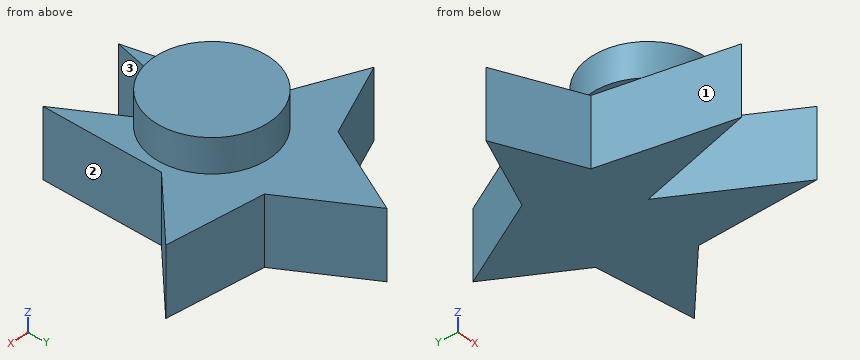
from build123d import *

# Parameters (mm, degrees)
F1_DEPTH = 35.306
F2_R     = 29.733819
F3_DEPTH = 17.526


with BuildPart() as f1:
    # F0 (on Top) → F1 (new body)
    with BuildSketch(Plane.XY):
        Polygon((-6.834473, 83.489791), (-29.494941, 37.89553), (-68.213977, 21.260617), (-28.555268, 3.504229), (-13.849725, -60.445834), (0, 0), (34.043796, -55.656485), (34.043796, 5.008644), (66.349685, 36.453225), (17.759997, 43.004174), align=None)
    extrude(amount=-F1_DEPTH)

    # F2 (on Top) → F3 (join)
    with BuildSketch(Plane.XY):
        Circle(F2_R)
    extrude(amount=F3_DEPTH)


solid = f1.part
Can you work these out from the model? Positions are in its coordinate system, mm. Face numbers are marked on the shaded views. A direction names the side the tool comes from. Give positions to 0.01 mm unless a question says otherwise; leave off trailing zeros. Loops run counter-clockwise (first coordinate to the right, second up) from the corner with the lowest first, then second, coordinate; pieces in that order, holes last. Notation, with made-up numbers: (46.5, -24.75) -> (50.5, -24.75) arc R17 ccw to (50.5, 5.25) -> close; hole circle Ø10 at (54, 78). An arc over 180 degrees is marked (long way). Return JSON: item names as keys, results as strings.
Q1. On a 3-axis mill with a long thin cutter (end or side, diameter ignored), from which of +Z, -Z, +X, -X, +Y, -Y can I reach the whole of each face in a straight line? I mean the marked faces 1, 2 and 3. Say none if no direction works.
Checks:
{"face 1": "-Z, -X, -Y", "face 2": "+Z, -Z, +X, -Y", "face 3": "-Z, -Y"}
Q2. I want a section at B-B, the plane y = -12. List the corners of the cut face in (x, z) for me.
Checks:
{"outline": "(-27.2, 0) -> (-24.99, 0) -> (-24.99, -35.31) -> (-2.75, -35.31) -> (-2.75, 0) -> (7.34, 0) -> (7.34, -35.31) -> (34.04, -35.31) -> (34.04, 0) -> (27.2, 0) -> (27.2, 17.53) -> (-27.2, 17.53) -> close"}
Q3. I need wall thicknesses on probe 1 along Z at (x, y) = (-17.5, 58); probe 2 along X at (y, z) = (-5, -20); probe 3 along Y at (x, z) = (0, 8). Which ranges of each line are inside material? Lowest first, please.
Checks:
{"probe 1": "z = -35.31 to 0", "probe 2": "x = -26.6 to -1.15, 3.06 to 34.04", "probe 3": "y = -29.73 to 29.73"}
Q4. For pin 1 Ø1 at (y, z) = (54, -21.5) entering from +X; pin 2 Ø4 at (y, z) = (-25.5, -7) entering from -X; pin 3 Ø3 at (x, z) = (-11, -26.5) entering from +Y, each with a flat end and sliding along its axis, tell me the tip position at first contact or that it passes through.
Checks:
{"pin 1": "stops at x = 11.38", "pin 2": "stops at x = -22.35", "pin 3": "stops at y = 78.13"}
Q5. I want a section at D-D, the plane y = -36. List the corners of the cut face in (x, z) for me, then the cut area to 3 significant figures.
Checks:
{"outline": "(-19.47, -35.31) -> (-8.25, -35.31) -> (-8.25, 0) -> (-19.47, 0) -> close; (22.02, -35.31) -> (34.04, -35.31) -> (34.04, 0) -> (22.02, 0) -> close", "area": "821 mm2"}
Q6. I want a section at C-C, the plane x = -10. List the corners of the cut face in (y, z) for me, then the cut area to 3 significant figures.
Checks:
{"outline": "(-43.64, -35.31) -> (77.12, -35.31) -> (77.12, 0) -> (28, 0) -> (28, 17.53) -> (-28, 17.53) -> (-28, 0) -> (-43.64, 0) -> close", "area": "5,250 mm2"}
Q7. I want a section at A-A, the plane z = -4.5. List the corners of the cut face in (x, y) for me.
Checks:
{"outline": "(-68.21, 21.26) -> (-28.56, 3.5) -> (-13.85, -60.45) -> (0, 0) -> (34.04, -55.66) -> (34.04, 5.01) -> (66.35, 36.45) -> (17.76, 43) -> (-6.83, 83.49) -> (-29.49, 37.9) -> close"}
